Model file for the job. Use its own axes, mm. Face numbers are marked on the shaded views. A direction names the side the tool comes from. Coordinates: 2 decimals unless noted, no trailing zeros. Loops run counter-clockwise (first coordinate to the right, second up) from the corner with the lowest first, then second, coordinate; pieces in that order, holes last. Notation, with made-up numbers: M 75.25,14.25 L 130.25,14.25 A20 ccw 130.25,46.25 Z; hole C -10.75,24 d2. An arc over 180 degrees is marked long. Write item = value, one per line. Start each with the question number.
from build123d import *

# Parameters (mm, degrees)
CROQUIS1_R                 = 1.5
CROQUIS1_R_2               = 2
CROQUIS1_R_3               = 4
SALIENTE_EXTRUIR1_DEPTH    = 2
CROQUIS2_W                 = 42
CROQUIS2_H                 = 2
CROQUIS2_W_2               = 8
SALIENTE_EXTRUIR2_DEPTH    = 25
REDONDEO2_R                = 2
CROQUIS3_R                 = 1.5
CROQUIS3_R_2               = 2
CORTAR_EXTRUIR1_DEPTH      = 25
CORTAR_EXTRUIR1_DEPTH_BACK = 25


with BuildPart() as part:
    # Croquis1 → Saliente-Extruir1 (new body)
    with BuildSketch(Plane.XY):
        with BuildLine():
            Line((-21, -12), (21, -12))
            Line((21, -12), (21, -5.5))
            Line((21, -5.5), (27, -5.5))
            ThreePointArc((27, -5.5), (28.414213562, -4.914213562), (29, -3.5))
            Line((29, -3.5), (29, 16.5))
            Line((29, 16.5), (21, 16.5))
            Line((21, 16.5), (21, 12.5))
            Line((21, 12.5), (19, 12.5))
            Line((19, 12.5), (19, 21.49))
            ThreePointArc((19, 21.49), (18.414213562, 22.904213562), (17, 23.49))
            Line((17, 23.49), (-17, 23.49))
            ThreePointArc((-17, 23.49), (-18.414213562, 22.904213562), (-19, 21.49))
            Line((-19, 21.49), (-19, 12.5))
            Line((-19, 12.5), (-21, 12.5))
            Line((-21, 12.5), (-21, 16.5))
            Line((-21, 16.5), (-29, 16.5))
            Line((-29, 16.5), (-29, -3.5))
            ThreePointArc((-29, -3.5), (-28.414213562, -4.914213562), (-27, -5.5))
            Line((-27, -5.5), (-21, -5.5))
            Line((-21, -5.5), (-21, -12))
        make_face()
        with Locations((0, 7)):
            Circle(CROQUIS1_R, mode=Mode.SUBTRACT)
        with Locations((7, 0)):
            Circle(CROQUIS1_R, mode=Mode.SUBTRACT)
        with Locations((0, -7)):
            Circle(CROQUIS1_R, mode=Mode.SUBTRACT)
        with Locations((-7, 0)):
            Circle(CROQUIS1_R, mode=Mode.SUBTRACT)
        with Locations((-24.25, 10.5)):
            Circle(CROQUIS1_R_2, mode=Mode.SUBTRACT)
        with Locations((24.25, 10.5)):
            Circle(CROQUIS1_R_2, mode=Mode.SUBTRACT)
        with Locations((-24.25, 0.5)):
            Circle(CROQUIS1_R_2, mode=Mode.SUBTRACT)
        Circle(CROQUIS1_R_3, mode=Mode.SUBTRACT)
        with Locations((10.5, 17.5)):
            Circle(CROQUIS1_R, mode=Mode.SUBTRACT)
        with Locations((17.5, 10.5)):
            Circle(CROQUIS1_R, mode=Mode.SUBTRACT)
        with Locations((10.5, 3.5)):
            Circle(CROQUIS1_R, mode=Mode.SUBTRACT)
        with Locations((3.5, 10.5)):
            Circle(CROQUIS1_R, mode=Mode.SUBTRACT)
        with Locations((-10.5, 17.5)):
            Circle(CROQUIS1_R, mode=Mode.SUBTRACT)
        with Locations((-3.5, 10.5)):
            Circle(CROQUIS1_R, mode=Mode.SUBTRACT)
        with Locations((-10.5, 3.5)):
            Circle(CROQUIS1_R, mode=Mode.SUBTRACT)
        with Locations((-17.5, 10.5)):
            Circle(CROQUIS1_R, mode=Mode.SUBTRACT)
        with Locations((-10.5, 10.5)):
            Circle(CROQUIS1_R_3, mode=Mode.SUBTRACT)
        with Locations((10.5, 10.5)):
            Circle(CROQUIS1_R_3, mode=Mode.SUBTRACT)
        with Locations((24.25, 0.5)):
            Circle(CROQUIS1_R_2, mode=Mode.SUBTRACT)
    extrude(amount=SALIENTE_EXTRUIR1_DEPTH)

    # Croquis2 → Saliente-Extruir2 (add)
    with BuildSketch(Plane.XY):
        with Locations((0, -13)):
            Rectangle(CROQUIS2_W, CROQUIS2_H)
        with Locations((-25, 17.5)):
            Rectangle(CROQUIS2_W_2, CROQUIS2_H)
        with Locations((25, 17.5)):
            Rectangle(CROQUIS2_W_2, CROQUIS2_H)
    extrude(amount=SALIENTE_EXTRUIR2_DEPTH)

    # Redondeo2
    redondeo2_edges = [part.edges().sort_by_distance(p)[0] for p in [
        (0, -14, 0),
        (-21, -13, 25),
        (21, -13, 25),
        (-25, 18.5, 0),
        (-21, 17.5, 25),
        (-29, 17.5, 25),
        (25, 18.5, 0),
        (29, 17.5, 25),
        (21, 17.5, 25),
    ]]
    fillet(redondeo2_edges, radius=REDONDEO2_R)

    # Croquis3 → Cortar-Extruir1 (cut, two sides)
    with BuildSketch(Plane(origin=(0, 0, 0), x_dir=(1, 0, 0), z_dir=(0, 1, 0))) as cortar_extruir1_sk:
        with Locations((-10.5, -12.5)):
            Circle(CROQUIS3_R)
        with Locations((10.5, -12.5)):
            Circle(CROQUIS3_R)
        with Locations((-10.5, -5.5)):
            Circle(CROQUIS3_R)
        with Locations((-3.5, -12.5)):
            Circle(CROQUIS3_R)
        with Locations((-10.5, -19.5)):
            Circle(CROQUIS3_R)
        with Locations((-17.5, -12.5)):
            Circle(CROQUIS3_R)
        with Locations((3.5, -12.5)):
            Circle(CROQUIS3_R)
        with Locations((10.5, -19.5)):
            Circle(CROQUIS3_R)
        with Locations((10.5, -5.5)):
            Circle(CROQUIS3_R)
        with Locations((17.5, -12.5)):
            Circle(CROQUIS3_R)
        with Locations((-25, -7.5)):
            Circle(CROQUIS3_R_2)
        with Locations((-25, -17.5)):
            Circle(CROQUIS3_R_2)
        with Locations((25, -17.5)):
            Circle(CROQUIS3_R_2)
        with Locations((25, -7.5)):
            Circle(CROQUIS3_R_2)
    extrude(amount=CORTAR_EXTRUIR1_DEPTH, mode=Mode.SUBTRACT)
    extrude(cortar_extruir1_sk.sketch, amount=-CORTAR_EXTRUIR1_DEPTH_BACK, mode=Mode.SUBTRACT)


solid = part.part
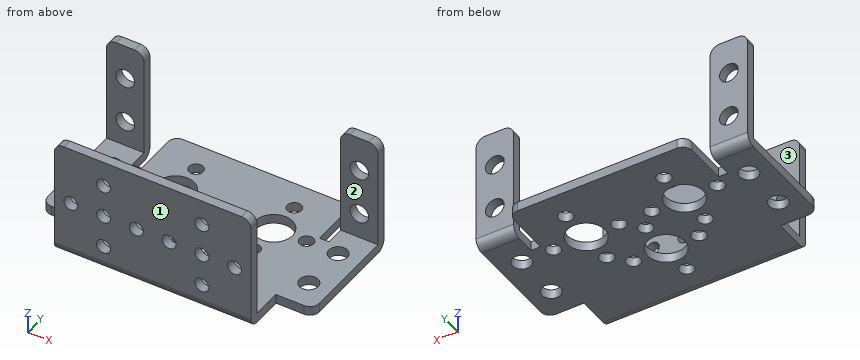
Item 1: Cut at A-A (z = 8.5). Give the cut face in (x, y), plus the area to 3 significant figures.
Item 2: Probe L1, parallel to Z at x = 10.5, y = -12.9; L2, parallel to Z at x = 10.5, y = -13; L3, parallel to Y at x = 24.25, z = 1.4. List the from-to ranges inside material, lowest first.
Item 3: Cut at C-C (y = 10.5). Give the number of separate pieces and of enclosed holes in the cut face, plus the area to 3 significant figures.
Item 4: Cut at B-B (x = 25). Give the cut face in (y, z), plus the area to 3 significant figures.
Item 5: 3-axis set-ups, long thin cutter, end or side, ignore diameter. For the marked faces 1, 2 and 3: which of +Z, -Z, +X, -X, +Y, -Y reach the whole face in a straight line?
Item 6: Pin check, flat tips, straight feed: pin 1 Ø2.5 at (x, y) = (0, 7) entering from -Z; pin 2 Ø3 at (x, z) = (22.5, 16) entering from +Y; pin 3 Ø2.5 at (x, z) = (24, 16) entering from -Y; pin 4 Ø1.6 at (x, z) = (25.5, 1.5) entering from -Y. Stop position of each tip, or through.
Reported:
q1.outline = M -29,16.5 L -26.73,16.5 L -26.73,18.5 L -29,18.5 Z; M -23.27,16.5 L -21,16.5 L -21,18.5 L -23.27,18.5 Z; M -21,-14 L 21,-14 L 21,-12 L -21,-12 Z; M 21,16.5 L 23.27,16.5 L 23.27,18.5 L 21,18.5 Z; M 26.73,16.5 L 29,16.5 L 29,18.5 L 26.73,18.5 Z
q1.area = 102 mm^2
q2.L1 = 0.21 to 4, 7 to 11, 14 to 18, 21 to 25
q2.L2 = 0.27 to 4, 7 to 11, 14 to 18, 21 to 25
q2.L3 = -5.5 to -1.5, 2.5 to 8.5, 12.5 to 18.41
q3.separate_pieces = 9
q3.enclosed_holes = 0
q3.area = 44.0 mm^2
q4.outline = M -5.5,0 L -1.35,0 L -1.35,2 L -5.5,2 Z; M 2.35,0 L 8.65,0 L 8.65,2 L 2.35,2 Z; M 12.35,0 L 16.5,0 A2 ccw 18.5,2 L 18.5,5.5 L 16.5,5.5 L 16.5,2 L 12.35,2 Z; M 16.5,9.5 L 18.5,9.5 L 18.5,15.5 L 16.5,15.5 Z; M 16.5,19.5 L 18.5,19.5 L 18.5,25 L 16.5,25 Z
q4.area = 62.3 mm^2
q5.face_1 = +Z, -Z, +X, -X, -Y
q5.face_2 = +Z, +X, -X, -Y
q5.face_3 = +Z, +X, -X, +Y
q6.pin_1 = through
q6.pin_2 = 18.5
q6.pin_3 = 16.5
q6.pin_4 = -5.5
